Work out the finished part from the listing and answer in its coordinate system (mm). A direction names the side the tool comes from. Coordinates: 2 decimals unless noted, no trailing zeros. Order: outer loops, then holes, each group sorted by start corner. A loop starts at its lowest first (then second) coordinate and runs counter-clockwise, first axis right, second up. Notation, with made-up numbers: (38, 84.25) - (46, 84.25) arc R30 ccw to (46, 108.25) - close; hole circle Ø9 at (28, -1). An arc over 180 degrees is marked (long way). Answer as a JSON object with one key per item and string values. Group by question number.
1) Section A-A (x = -48) is taken. Give the vertices of the cut face in (y, z).
2) Section B-B (y = 34.5) is taken. Give the vertices of the cut face in (x, z).
3) A tool of negligible diameter and unlimited length cuts with its end or side. For faces 4 (the face through (-54, 39, 0)), 5 (the face through (-52.125, 30.649, 18.961)), from which of +Z, -Z, +X, -X, +Y, -Y can it reach the whole face along a straight path? Write none if from no direction.
4) Each of these flat-tipped pins is pushed along its axis until it touches: P1, Ø2, axis at y = 38, z = 18, coming from the +X side; P2, Ø6, axis at y = 40.5, z = 21.5, coming from the +X side. Where does it stop, or does it pass through?
5) Section D-D (z = 9) is taken. Give the vertices of the cut face in (x, y), plus the area to 3 significant figures.
6) Find the intervals of material crossed by line 1 along Y through (x, z) = (-41.5, 8); line 2 along Z through (x, y) = (-62.5, 44); line 3 along X through (y, z) = (40.5, 1.75), in increasing order.
7) The mould has two halves that part along Y. Classify faces 1 (the face through (-61.875, 52.618, 6.439)), 2 (the face through (-33.545, 38, 6)), 3 (the face through (-50, 60.125, 6)): released by +Y, released by -Y, zero draft, split by the parting line, or undercut.
8) Section C-C (x = -42) is taken. Give the vertices of the cut face in (y, z), plus the area to 3 significant figures.
from build123d import *

# Parameters (mm, degrees)
F0_W      = 32.445639
F0_H      = 43.444172
F1_DEPTH  = 12.7
F2_R      = 8.464038
F3_DEPTH  = 12.7
F4_R      = 7.201961
F5_DEPTH  = 25.4
F8_R      = 3.287286
F9_DEPTH  = 25.4
F10_R     = 2.865858
F11_DEPTH = 25.4
F12_R     = 3.833987
F13_DEPTH = 25.4


with BuildPart() as f1:
    # F0 (on Top) → F1 (new body)
    with BuildSketch(Plane.XY):
        with Locations((-49.768306, 38.403161)):
            Rectangle(F0_W, F0_H)
    extrude(amount=F1_DEPTH)

    # F2 (on face) → F3 (join)
    with BuildSketch(Plane.XY.offset(12.7)):
        with Locations((-45.408141, 35.799652)):
            Circle(F2_R)
    extrude(amount=F3_DEPTH)

    # F4 (on face) → F5 (cut)
    with BuildSketch(Plane.XY.offset(25.4)):
        with Locations((-45.408141, 35.799652)):
            Circle(F4_R)
    extrude(amount=-F5_DEPTH, mode=Mode.SUBTRACT)

    # F8 (on face) → F9 (cut)
    with BuildSketch(Plane.XY.offset(12.7)):
        with Locations((-58.590725, 52.473925)):
            Circle(F8_R)
    extrude(amount=-F9_DEPTH, mode=Mode.SUBTRACT)

    # F10 (on face) → F11 (cut)
    with BuildSketch(Plane.XY.offset(12.7)):
        with Locations((-39.644916, 54.891884)):
            Circle(F10_R)
    extrude(amount=-F11_DEPTH, mode=Mode.SUBTRACT)

    # F12 (on face) → F13 (cut)
    with BuildSketch(Plane.XY.offset(12.7)):
        with Locations((-59.598204, 23.901373)):
            Circle(F12_R)
    extrude(amount=-F13_DEPTH, mode=Mode.SUBTRACT)


solid = f1.part
Report:
{
 "1": {"outline": "(16.68, 0) - (29.08, 0) - (29.08, 25.4) - (27.74, 25.4) - (27.74, 12.7) - (16.68, 12.7) - close; (42.52, 0) - (60.13, 0) - (60.13, 12.7) - (43.86, 12.7) - (43.86, 25.4) - (42.52, 25.4) - close"},
 "2": {"outline": "(-65.99, 0) - (-52.49, 0) - (-52.49, 25.4) - (-53.77, 25.4) - (-53.77, 12.7) - (-65.99, 12.7) - close; (-38.32, 0) - (-33.55, 0) - (-33.55, 12.7) - (-37.04, 12.7) - (-37.04, 25.4) - (-38.32, 25.4) - close"},
 "3": {"face 4": "-Z, +X, -X, +Y, -Y", "face 5": "+Z"},
 "4": {"P1": "stops at x = -37.03", "P2": "stops at x = -37.12"},
 "5": {"outline": "(-65.99, 16.68) - (-33.55, 16.68) - (-33.55, 60.13) - (-65.99, 60.13) - close; hole circle Ø7.67 at (-59.6, 23.9); hole circle Ø6.57 at (-58.59, 52.47); hole circle Ø14.4 at (-45.41, 35.8); hole circle Ø5.73 at (-39.64, 54.89)", "area": "1,140 mm²"},
 "6": {"line 1": "y = 16.68 to 29.75, 41.85 to 52.71, 57.08 to 60.13", "line 2": "z = 0 to 12.7", "line 3": "x = -65.99 to -50.86, -39.95 to -33.55"},
 "7": {"face 1": "undercut", "face 2": "zero draft", "face 3": "released by +Y"},
 "8": {"outline": "(16.68, 0) - (29.46, 0) - (29.46, 25.4) - (28.05, 25.4) - (28.05, 12.7) - (16.68, 12.7) - close; (42.14, 0) - (53.26, 0) - (53.26, 12.7) - (43.55, 12.7) - (43.55, 25.4) - (42.14, 25.4) - close; (56.52, 0) - (60.13, 0) - (60.13, 12.7) - (56.52, 12.7) - close", "area": "385 mm²"}
}
